The drawing under review shows one solid part. Ordinate dimensions are in mm from its lowest x, y, z. Round coordinates to 2 decimals unless told otherwise and drop trailing zeros. Loops run counter-clockwise (first coordinate to the right, second up) from the corner with the lowest first, then second, coordinate; pieces in that order, holes last. Notation, with made-up numbers: (-22.5, 52.5) -> (-2.5, 52.5) arc R32 ccw to (-2.5, 82.5) -> close; hole circle Ø10 at (-24.5, -14.5). An arc over 180 degrees is marked (long way). Use a Markdown table: item, result. Add a question column.
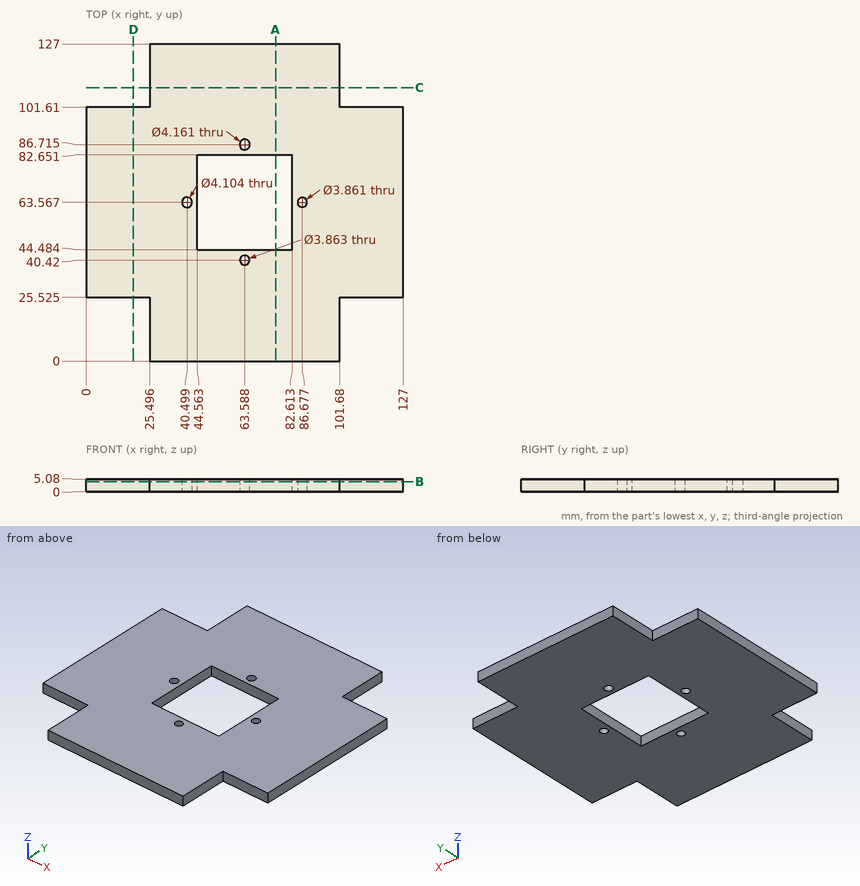
1. Consider section A-A on x = 76. State the section outline as (y, z) points, plus the area to 3 significant figures.
2. Consider section B-B on z = 4. Give the number of separate pieces and of enclosed holes in the cut face, plus the area to 3 significant figures.
3. To check wall thickness, follow probe 1 along X at (y, z) = (58, 4.65); probe 2 along Y at (x, z) = (68, 4.4); probe 3 along Y at (x, z) = (108, 0.85) (1 decimal). State the ranges of each line that lie inside material, in increasing order. Write a range as from..to.
4. Consider section D-D on x = 19. State the section outline as (y, z) points (1 decimal).
5. Insertion check: P1, Ø3, axis at y = 95, z = 2.5, coming from the -X side; P2, Ø1.5, axis at y = 109.5, z = 3, coming from the +X side. Each pin has a flat end and moves straight along its axis. Give the tip position at first contact, or say it passes through.
6. Consider section C-C on y = 109.5. State the section outline as (x, z) points.
Verdict:
| question | item | result |
|---|---|---|
| 1 | outline | (0, 0) -> (44.48, 0) -> (44.48, 5.08) -> (0, 5.08) -> close; (82.65, 0) -> (127, 0) -> (127, 5.08) -> (82.65, 5.08) -> close |
| 1 | area | 451 mm² |
| 2 | separate pieces | 1 |
| 2 | enclosed holes | 5 |
| 2 | area | 12,000 mm² |
| 3 | probe 1 | x = 0..44.56, 82.61..127 |
| 3 | probe 2 | y = 0..44.48, 82.65..127 |
| 3 | probe 3 | y = 25.5..101.6 |
| 4 | outline | (25.5, 0) -> (101.6, 0) -> (101.6, 5.1) -> (25.5, 5.1) -> close |
| 5 | P1 | stops at x = 0 |
| 5 | P2 | stops at x = 101.68 |
| 6 | outline | (25.5, 0) -> (101.68, 0) -> (101.68, 5.08) -> (25.5, 5.08) -> close |
